CAD build for the part. Positions are in the model's coordinates, mm. Face numbers are marked on the shaded views. A direction names the side the tool comes from. Coordinates: 2 decimals unless noted, no trailing zeros. Loops run counter-clockwise (first coordinate to the right, second up) from the corner with the lowest first, then second, coordinate; pieces in that order, holes last. Notation, with made-up numbers: (12.5, 30) - (48.5, 30) arc R14 ccw to (48.5, 51) - close; hole circle Ø5 at (26, 81.25). An arc over 180 degrees is marked (long way). Put each result on its own line as item: value.
```python
from build123d import *

# Parameters (mm, degrees)
SKETCH1_W           = 152.4
SKETCH1_H           = 12.7
EXTRUDE_THIN1_DEPTH = 6.35
FILLET1_R           = 2.54
SKETCH3_R           = 1.651
CUT_EXTRUDE1_DEPTH  = 6.35
LPATTERN1_COUNT     = 2
LPATTERN1_PITCH     = 144.78
SKETCH4_W           = 147.32
SKETCH4_H           = 2.54
EXTRUDE_THIN2_DEPTH = 31.75
CUT_EXTRUDE2_DEPTH  = 2.54
FILLET2_R           = 2.54
SKETCH7_R           = 1.651
CUT_EXTRUDE3_DEPTH  = 2.54


with BuildPart() as part:
    # Sketch1 → Extrude-Thin1 (new body)
    with BuildSketch(Plane(origin=(0, 0, 0), x_dir=(1, 0, 0), z_dir=(0, 1, 0))):
        with Locations((0, -6.35)):
            Rectangle(SKETCH1_W, SKETCH1_H)
    extrude(amount=EXTRUDE_THIN1_DEPTH)

    # Fillet1
    fillet1_edges = [part.edges().sort_by_distance(p)[0] for p in [
        (-76.2, 3.175, 12.7),
        (-76.2, 3.175, 0),
        (76.2, 3.175, 0),
        (76.2, 3.175, 12.7),
    ]]
    fillet(fillet1_edges, radius=FILLET1_R)

    # Sketch3 → Cut-Extrude1 (cut)
    with BuildSketch(Plane(origin=(0, 6.35, 0), x_dir=(1, 0, 0), z_dir=(0, 1, 0))):
        with Locations((72.520050335, -6.35)):
            Circle(SKETCH3_R)
    cut_extrude1 = extrude(amount=-CUT_EXTRUDE1_DEPTH, mode=Mode.SUBTRACT)

    # LPattern1: Cut-Extrude1 ×2
    with Locations(*[(-i * LPATTERN1_PITCH, 0, 0) for i in range(1, LPATTERN1_COUNT)]):
        add(cut_extrude1, mode=Mode.SUBTRACT)

    # Sketch4 → Extrude-Thin2 (add)
    with BuildSketch(Plane.XY.offset(12.7)):
        with Locations((0, 1.27)):
            Rectangle(SKETCH4_W, SKETCH4_H)
    extrude(amount=EXTRUDE_THIN2_DEPTH)

    # Sketch5 → Cut-Extrude2 (cut)
    with BuildSketch(Plane(origin=(0, 0, 0), x_dir=(-1, 0, 0), z_dir=(0, -1, 0))):
        Polygon((-73.66, -12.7), (-58.727381013, -12.7), (-73.66, -36.704605771), align=None)
    cut_extrude2 = extrude(amount=-CUT_EXTRUDE2_DEPTH, mode=Mode.SUBTRACT)

    # Mirror1: Cut-Extrude2 across plane
    add(cut_extrude2.mirror(Plane(origin=(0, 0, 0), x_dir=(0, 0, 1), z_dir=(1, 0, 0))), mode=Mode.SUBTRACT)

    # Fillet2
    fillet2_edges = [part.edges().sort_by_distance(p)[0] for p in [
        (-73.66, 1.27, 36.704605771),
        (73.66, 1.27, 44.45),
        (-73.66, 1.27, 44.45),
        (73.66, 1.27, 36.704605771),
    ]]
    fillet(fillet2_edges, radius=FILLET2_R)

    # Sketch7 → Cut-Extrude3 (cut)
    with BuildSketch(Plane(origin=(0, 2.54, 0), x_dir=(1, 0, 0), z_dir=(0, 1, 0))):
        with Locations((-69.342, -40.386)):
            Circle(SKETCH7_R)
    cut_extrude3 = extrude(amount=-CUT_EXTRUDE3_DEPTH, mode=Mode.SUBTRACT)

    # Mirror2: Cut-Extrude3 across plane
    add(cut_extrude3.mirror(Plane(origin=(0, 0, 0), x_dir=(0, 0, 1), z_dir=(1, 0, 0))), mode=Mode.SUBTRACT)


solid = part.part
```
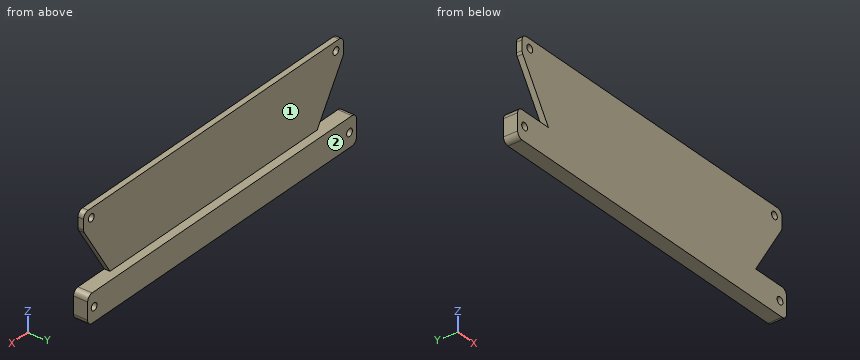
Q1. Wall check: L1, parallel to X at y = 3.25, z = 6.35; L2, parallel to X at y = 1.25, z = 5.5; L3, parallel to Y at x = -10.5, z = 23.5. Give the ranges that are in metal, low to high. Write a range as from..to.
Determined:
L1: -76.2..-73.91, -70.61..70.87, 74.17..76.2
L2: -76.2..-73.68, -70.84..71.1, 73.94..76.2
L3: 0..2.54
Q2. Slice it at C-C, the plane y = 1.5. Give the cut face in (x, z), then the cut area to 3 significant figures.
Determined:
outline: (-76.2, 2.54) arc R2.54 ccw to (-73.66, 0) - (73.66, 0) arc R2.54 ccw to (76.2, 2.54) - (76.2, 10.16) arc R2.54 ccw to (73.66, 12.7) - (58.73, 12.7) - (73.28, 36.09) arc R2.54 ccw to (73.66, 37.43) - (73.66, 41.91) arc R2.54 ccw to (71.12, 44.45) - (-71.12, 44.45) arc R2.54 ccw to (-73.66, 41.91) - (-73.66, 37.43) arc R2.54 ccw to (-73.28, 36.09) - (-58.73, 12.7) - (-73.66, 12.7) arc R2.54 ccw to (-76.2, 10.16) - close; hole circle Ø3.3 at (-72.26, 6.35); hole circle Ø3.3 at (-69.34, 40.39); hole circle Ø3.3 at (69.34, 40.39); hole circle Ø3.3 at (72.52, 6.35)
area: 6,210 mm2
Q3. Slice it at B-B, the plane x = 63.5. Give the cut face in (y, z), then the cut area to 3 significant figures.
Determined:
outline: (0, 0) - (6.35, 0) - (6.35, 12.7) - (0, 12.7) - close; (0, 20.37) - (2.54, 20.37) - (2.54, 44.45) - (0, 44.45) - close
area: 142 mm2
Q4. Slice it at A-A, the plane z = 6.35. Give the cut face in (x, y).
Determined:
outline: (-76.2, 0) - (-73.91, 0) - (-73.91, 6.35) - (-76.2, 6.35) - close; (-70.61, 0) - (70.87, 0) - (70.87, 6.35) - (-70.61, 6.35) - close; (74.17, 0) - (76.2, 0) - (76.2, 6.35) - (74.17, 6.35) - close
Q5. Pin check, flat tips, straight feed: pin 1 Ø4 at (x, z) = (72.52, 6.35) entering from -Y; pin 2 Ø4.5 at (x, z) = (69.342, 40.386) entering from +Y; pin 3 Ø3 at (y, z) = (1, 40.5) entering from +X; pin 4 Ø1.5 at (y, z) = (2.5, 30.5) entering from +X. Stop position of each tip, or through.
Determined:
pin 1: y = 0
pin 2: y = 2.54
pin 3: x = 73.66
pin 4: x = 70.27
Q6. Tool access for the marked faces 1 and 2: list every direction of +Z, -Z, +X, -X, +Y, -Y with a clear straight run to the whole face (end or side of a thin tool).
Determined:
face 1: +Z, +X, -X, +Y
face 2: +Z, -Z, +X, -X, +Y
Q7. Slice it at D-D, the plane x = 24. Give the cut face in (y, z).
Determined:
outline: (0, 0) - (6.35, 0) - (6.35, 12.7) - (2.54, 12.7) - (2.54, 44.45) - (0, 44.45) - close
